Verification items for the finished model (mm, model axes). A direction names the side the tool comes from. Coordinates: 2 decimals unless noted, no trailing zeros. Write each loop counter-clockwise with the first axis right and the second up, starting at its lowest first coordinate (ties: lowest second). Pieces come first, ordered by that corner, then holes. Notation, with made-up numbers: (89.25, 76) -> (102.25, 76) arc R24 cw to (102.25, 113) -> close; hole circle Ø4 at (24.25, 10.5). An arc over 180 degrees is marked (long way). Answer in a Markdown table with one row per item.
Autodesk Fusion 360 part; units mm, degrees
sketch "Sketch1" plane through (0, 0, 0) normal (0, 0, 1) x (1, 0, 0)
  line L0 (72.4034, 27.9167) -> (178.4034, 27.9167)
  line L1 (72.4034, 27.9167) -> (72.4034, 39.1667)
  line L2 (72.4034, 39.1667) -> (28.4034, 39.1667)
  line L3 (28.4034, 39.1667) -> (28.4034, 60.6444)
  line L4 (51.7694, 73.8535) -> (80.618, 84.3536) construction
  line L5 (51.7694, 73.8535) -> (87.8768, 73.8535) construction
  line L6 (80.618, 84.3536) -> (22.8269, 63.3193) construction
  line L7 (80.618, 84.3536) -> (137.5254, 84.3536) construction
  line L8 (178.4034, 73.4926) -> (77.2668, 73.4926)
  line L9 (72.4034, 39.1667) -> (72.4034, 27.9167)
  arc A0 (178.4034, 37.4167) -> (178.4034, 63.4167) centre (178.4034, 50.4167) ccw
  line L10 (178.4034, 27.9167) -> (178.4034, 37.4167)
  line L11 (178.4034, 63.4167) -> (178.4034, 73.4926)
  line L12 (0, 0) -> (200, 0)
  line L13 (200, 0) -> (200, 115)
  line L14 (200, 115) -> (0, 115)
  line L15 (0, 115) -> (0, 0)
  circle A1 centre (80.618, 84.3536) radius 2.5
  circle A2 centre (22.8269, 63.3193) radius 2.5
  line L16 (178.4034, 73.4926) -> (178.4034, 27.9167) construction
  line L17 (178.4034, 50.4167) -> (28.4034, 50.4167)
  line L18 (75.7554, 82.5838) -> (66.8629, 107.0158)
  line L19 (75.7554, 82.5838) -> (66.8629, 107.0158)
  line L20 (66.8629, 107.0158) -> (17.9989, 89.2307)
  line L21 (17.9989, 89.2307) -> (26.8914, 64.7987)
  line L22 (75.7554, 82.5838) -> (75.7337, 82.5692)
  arc A3 (77.2668, 73.4926) -> (75.7316, 82.5751) centre (51.7694, 73.8535) ccw
  line L23 (26.8914, 64.7987) -> (28.4034, 60.6444)
  dimension "d3" = 106
  dimension "d5" = 26
  dimension "d8" = 11.25
  dimension "d9" = 44
  dimension "d11" = 30.7
  dimension "d12" = 20
  dimension "d14" = 61.5
  dimension "d15" = 200
  dimension "d16" = 115
  dimension "d17" = 5
  dimension "d18" = 5
  dimension "d27" = 26
  dimension "d28" = 26
  dimension "d29" = 52
extrude "Extrude3" add sketch "Sketch1" along normal blind 6
fillet "Fillet3" radius 3 1 edges at (200, 0, 3)
fillet "Fillet4" radius 3 3 edges at (0, 0, 3) (0, 115, 3) (200, 115, 3)
fillet "Fillet5" radius 2 7 edges at (17.9989, 89.2307, 3) (66.8629, 107.0158, 3) (77.2668, 73.4926, 3) (28.4034, 39.1667, 3) (72.4034, 27.9167, 3) (178.4034, 27.9167, 3) (178.4034, 73.4926, 3)
fillet "Fillet6" radius 2 1 edges at (72.4034, 39.1667, 3)
1. Thickness scan on line 1 (X direction, y = 31.5, z = 3.85); line 2 (X direction, y = 50, z = 3.2); line 3 (Y direction, x = 85, z = 5.1). Record the ranges inside material, lowest first. Write a range as from..to.
Geometry says:
| item | result |
|---|---|
| line 1 | 0..72.4, 178.4..200 |
| line 2 | 0..28.4, 191.4..200 |
| line 3 | 0..27.92, 73.49..115 |
2. Mould release check, pull along Y, two halves, no side actions. Record for faces 3 (the flat face through (128, 73.493, 3)), 4 (the flat face through (99, 0, 3)), 5 (the flat face through (200, 57, 3)): released by +Y, released by -Y, zero draft, split by the parting line, or undercut.
Geometry says:
| item | result |
|---|---|
| face 3 | undercut |
| face 4 | released by -Y |
| face 5 | zero draft |
3. Section check C-C, the plane z = 4.95. State how many separate pieces and enclosed holes the cut face has, plus the area to 3 significant figures.
Geometry says:
| item | result |
|---|---|
| separate pieces | 1 |
| enclosed holes | 3 |
| area | 15,000 mm^2 |
4. Section check B-B, the plane y = 77.5. Record the boundary of the cut face in (x, z), plus the area to 3 significant figures.
Geometry says:
| item | result |
|---|---|
| outline | (0, 0) -> (22.27, 0) -> (22.27, 6) -> (0, 6) -> close; (77.01, 0) -> (200, 0) -> (200, 6) -> (77.01, 6) -> close |
| area | 872 mm^2 |
5. Tool access check on faces 1 (the flat face through (125, 27.917, 3)), 2 (the flat face through (99, 84, 0)). Record the directions out of +Z, -Z, +X, -X, +Y, -Y that give a thin tool (end or side, any length) a straight path to the whole face; none if there is none.
Geometry says:
| item | result |
|---|---|
| face 1 | +Z, -Z |
| face 2 | -Z, +X, -X, +Y, -Y |
6. Section check A-A, the plane x = 154. Record the boundary of the cut face in (y, z).
Geometry says:
| item | result |
|---|---|
| outline | (0, 0) -> (27.92, 0) -> (27.92, 6) -> (0, 6) -> close; (73.49, 0) -> (115, 0) -> (115, 6) -> (73.49, 6) -> close |
